```python
from build123d import *

# Parameters (mm, degrees)
SZKIC1_W                             = 150
SZKIC1_H                             = 100
DODANIE_WYCI_GNI_CIE1_DEPTH          = 4
OTW_R_POD_RUB_M101_D                 = 11
LUSTRO1_AT_THE_SECOND_PLANE_COPY_1_D = 11


with BuildPart() as part:
    # Szkic1 → Dodanie-wyciągnięcie1 (new body)
    with BuildSketch(Plane.XY):
        Rectangle(SZKIC1_W, SZKIC1_H)
    extrude(amount=DODANIE_WYCI_GNI_CIE1_DEPTH)

    # Otwór pod śrubę M101 (through all)
    with Locations(Plane.XY.offset(4)):
        with Locations((-63, 38)):
            otw_r_pod_rub_m101 = Hole(OTW_R_POD_RUB_M101_D / 2)

    # Lustro1: Otwór pod śrubę M101 across plane
    add(otw_r_pod_rub_m101.mirror(Plane.ZX), mode=Mode.SUBTRACT)

    # Lustro1 at the second plane: Otwór pod śrubę M101 across plane
    add(otw_r_pod_rub_m101.mirror(Plane(origin=(0, 0, 0), x_dir=(0, 0, 1), z_dir=(1, 0, 0))), mode=Mode.SUBTRACT)

    # Lustro1 at the second plane copy 1 (through all)
    with Locations(Plane(origin=(0, 0, 4), x_dir=(-1, 0, 0), z_dir=(0, 0, 1))):
        with Locations((-63, 38)):
            Hole(LUSTRO1_AT_THE_SECOND_PLANE_COPY_1_D / 2)


solid = part.part
```
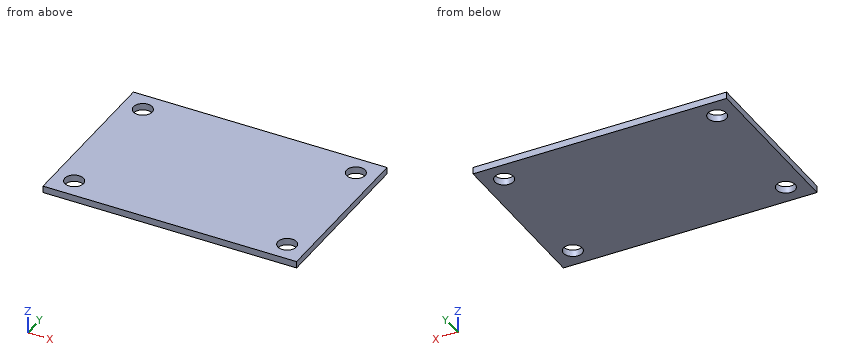
Work out the finished part from the listing and answer in its coordinate system (mm). Round coordinates to 2 decimals unless told otherwise and drop trailing zeros. Loops run counter-clockwise (first coordinate to the right, second up) from the corner with the lowest first, then second, coordinate; pieces in that order, holes last. Notation, with made-up numbers: M -3.75,70.5 L 46.25,70.5 A20 cw 46.25,92.5 Z; hole C -10,57 d11. An arc over 180 degrees is marked long. One line per question, with ' | ' between items.
Q1. This flat-tipped pin is pushed along its axis until it touches: pin 1 Ø9 at (x, y) = (-63, -38) entering from +Z. Where does it stop, or does it pass through?
Conclusion:
pin 1: passes through
Q2. Find section B-B, the plane y = -38. Give the vertices of the cut face in (x, z).
Conclusion:
outline: M -75,0 L -68.5,0 L -68.5,4 L -75,4 Z; M -57.5,0 L 57.5,0 L 57.5,4 L -57.5,4 Z; M 68.5,0 L 75,0 L 75,4 L 68.5,4 Z
Q3. Find section C-C, the plane z = 0.85. Give the vertices of the cut face in (x, y).
Conclusion:
outline: M -75,-50 L 75,-50 L 75,50 L -75,50 Z; hole C -63,-38 d11; hole C -63,38 d11; hole C 63,-38 d11; hole C 63,38 d11
Q4. Consider line 1 along Y through (x, z) = (-63, 2.7); line 2 along X through (y, z) = (-37.5, 3.4); line 3 along Y through (x, z) = (66, 0.3). Determine where each line is inside the solid, lowest interval first. Write a range as from..to.
Conclusion:
line 1: y = -50..-43.5, -32.5..32.5, 43.5..50 | line 2: x = -75..-68.48, -57.52..57.52, 68.48..75 | line 3: y = -50..-42.61, -33.39..33.39, 42.61..50
Q5. Find section A-A, the plane x = 63. Give the vertices of the cut face in (y, z), then the cut area to 3 significant figures.
Conclusion:
outline: M -50,0 L -43.5,0 L -43.5,4 L -50,4 Z; M -32.5,0 L 32.5,0 L 32.5,4 L -32.5,4 Z; M 43.5,0 L 50,0 L 50,4 L 43.5,4 Z | area: 312 mm2
